from build123d import *

# Parameters (mm, degrees)
SKETCH1_R           = 13.5
BOSS_EXTRUDE1_DEPTH = 15
SHELL1_T            = -1.5
SKETCH2_R           = 4.1
CUT_EXTRUDE1_DEPTH  = 20
BOSS_EXTRUDE2_START = 6
SKETCH3_R           = 6.1
SKETCH3_R_2         = 4.1
BOSS_EXTRUDE2_DEPTH = 6
SKETCH4_R           = 15
SKETCH4_R_2         = 12.5
BOSS_EXTRUDE3_DEPTH = 2


with BuildPart() as part:
    # Sketch1 → Boss-Extrude1 (new body)
    with BuildSketch(Plane(origin=(0, 0, 0), x_dir=(1, 0, 0), z_dir=(0, 1, 0))):
        with Locations(Location((0, 0, 0), (0, 0, 270))):
            Circle(SKETCH1_R)
    extrude(amount=BOSS_EXTRUDE1_DEPTH)

    # Shell1
    shell1_openings = [part.faces().sort_by_distance(p)[0] for p in [
        (0, 15, 0),
    ]]
    offset(amount=SHELL1_T, openings=shell1_openings, kind=Kind.INTERSECTION)

    # Sketch2 → Cut-Extrude1 (cut)
    with BuildSketch(Plane(origin=(0, 1.5, 0), x_dir=(1, 0, 0), z_dir=(0, 1, 0))):
        with Locations(Location((0, 0, 0), (0, 0, 270))):
            Circle(SKETCH2_R)
    extrude(amount=-CUT_EXTRUDE1_DEPTH, mode=Mode.SUBTRACT)

    # Sketch3 → Boss-Extrude2 (add)
    with BuildSketch(Plane(origin=(0, 1.5, 0), x_dir=(1, 0, 0), z_dir=(0, 1, 0)).offset(BOSS_EXTRUDE2_START)):
        with Locations(Location((0, 0, 0), (0, 0, 90))):
            Circle(SKETCH3_R)
        with Locations(Location((0, 0, 0), (0, 0, 270))):
            Circle(SKETCH3_R_2, mode=Mode.SUBTRACT)
    extrude(amount=-BOSS_EXTRUDE2_DEPTH)


with BuildPart() as body_2:
    # Sketch4 → Boss-Extrude3 (new body)
    with BuildSketch(Plane.XZ):
        with Locations(Location((0, 0, 0), (0, 0, 270))):
            Circle(SKETCH4_R)
        with Locations(Location((0, 0, 0), (0, 0, 270))):
            Circle(SKETCH4_R_2, mode=Mode.SUBTRACT)
    extrude(amount=-BOSS_EXTRUDE3_DEPTH)


with BuildPart() as part_1:
    add(part.part)

    # Combine1: union body 2
    add(body_2.part)


solid = part_1.part
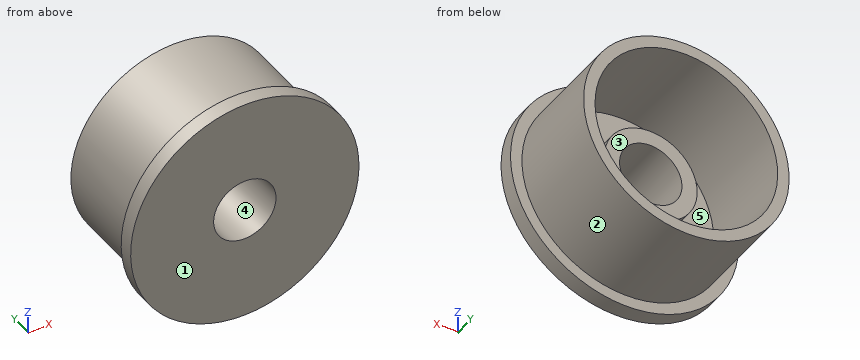
Build history of the part. All positions in model axes, mm. Face numbers are marked on the shaded views. A direction names the side the tool comes from. Give positions to 0.01 mm unless a question says otherwise; leave off trailing zeros. Order: outer loops, then holes, each group sorted by start corner. A loop starts at its lowest first (then second) coordinate and runs counter-clockwise, first axis right, second up. Notation, with made-up numbers: M 80,-7.75 L 95,-7.75 A20 cw 95,8.25 Z; hole C -27.75,38.5 d4. An arc over 180 degrees is marked long. Put each result on its own line as item: value.
Item 1: Flat gauge pins, fed straight in: pin 1 Ø6 at (x, y) = (6.5, 2) entering from +Z; pin 2 Ø3 at (x, y) = (-5.5, 3) entering from +Z; pin 3 Ø6 at (y, z) = (7.5, 2) entering from +X; pin 4 Ø5 at (x, z) = (0, 0) entering from +Y. Where does each tip first touch, or does it go through?
From the geometry:
pin 1: stops at z = 14.59
pin 2: stops at z = 14.35
pin 3: stops at x = 13.5
pin 4: passes through
Item 2: Slice it at D-D, the plane z = -5.5. Write the cut outline in (x, y).
From the geometry:
outline: M -13.96,0 L 13.96,0 L 13.96,2 L 12.33,2 L 12.33,15 L 10.67,15 L 10.67,1.5 L 2.64,1.5 L 2.64,7.5 L -2.64,7.5 L -2.64,1.5 L -10.67,1.5 L -10.67,15 L -12.33,15 L -12.33,2 L -13.96,2 Z
Item 3: Slice it at A-A, the plane z = 0. Write the cut outline in (x, y).
From the geometry:
outline: M -15,0 L -4.1,0 L -4.1,7.5 L -6.1,7.5 L -6.1,1.5 L -12,1.5 L -12,15 L -13.5,15 L -13.5,2 L -15,2 Z; M 4.1,0 L 15,0 L 15,2 L 13.5,2 L 13.5,15 L 12,15 L 12,1.5 L 6.1,1.5 L 6.1,7.5 L 4.1,7.5 Z
Item 4: Slice it at C-C, the plane y = 6.5. Write the cut outline in (x, z), plus the area to 3 significant figures.
From the geometry:
outline: C 0,0 d27; C 0,0 d12.2; hole C 0,0 d24; hole C 0,0 d8.2
area: 184 mm2
Item 5: Probe line 1 (X direction, y = 6.5, z = 0); line 2 (X direction, y = 9, z = 0); line 3 (Y direction, x = -9.25, z = -2.5). List the from-to ranges inside material, lowest first. Write a range as [from, to].
From the geometry:
line 1: x = [-13.5, -12], [-6.1, -4.1], [4.1, 6.1], [12, 13.5]
line 2: x = [-13.5, -12], [12, 13.5]
line 3: y = [0, 1.5]
Item 6: Two-plate mould, pull along X, no slides. Class the marked faces 1, 2 and 3: +X half, -X half, draft (parallel to the pull), parting line (faces both ways), or undercut.
From the geometry:
face 1: draft
face 2: parting line
face 3: undercut
Item 7: Slice it at B-B, the plane x = 0. Write the cut outline in (y, z).
From the geometry:
outline: M 0,-15 L 2,-15 L 2,-13.5 L 15,-13.5 L 15,-12 L 1.5,-12 L 1.5,-6.1 L 7.5,-6.1 L 7.5,-4.1 L 0,-4.1 Z; M 0,4.1 L 7.5,4.1 L 7.5,6.1 L 1.5,6.1 L 1.5,12 L 15,12 L 15,13.5 L 2,13.5 L 2,15 L 0,15 Z
Item 8: 3-axis set-ups, long thin cutter, end or side, ignore diameter. For the marked faces 4 and 5: which of +Z, -Z, +X, -X, +Y, -Y reach the whole face in a straight line?
From the geometry:
face 4: +Y, -Y
face 5: +Y
